CAD build for the part. Positions are in the model's coordinates, mm. A direction names the side the tool comes from. Give positions to 0.01 mm unless a question says otherwise; leave off trailing zeros. Loops run counter-clockwise (first coordinate to the right, second up) from the corner with the lowest first, then second, coordinate; pieces in that order, holes last.
```python
from build123d import *

# Parameters (mm, degrees)
RESSALTO_EXTRUS_O1_DEPTH = 6
CORTE_EXTRUS_O1_DEPTH    = 3.1
ESBO_O4_R                = 15
CORTE_EXTRUS_O2_DEPTH    = 100.844211363
ESBO_O6_R                = 2
CORTE_EXTRUS_O3_DEPTH    = 3.1
CORTE_EXTRUS_O7_DEPTH    = 10


with BuildPart() as part:
    # Esboço2 → Ressalto-extrusão1 (new body)
    with BuildSketch(Plane.XY):
        Polygon((70.472925804, 27.825776133), (30.15608873, 69.507678721), (-27.825776133, 70.472925804), (-69.507678721, 30.15608873), (-70.472925804, -27.825776133), (-30.15608873, -69.507678721), (27.825776133, -70.472925804), (69.507678721, -30.15608873), align=None)
    extrude(amount=RESSALTO_EXTRUS_O1_DEPTH)

    # Esboço3 → Corte-extrusão1 (cut)
    with BuildSketch(Plane.XY.offset(6)):
        Polygon((-61.0871998, -37.529288249), (-39.534791939, -59.811427182), (-25.159218434, -45.906647917), (-46.711626295, -23.624508984), align=None)
        Polygon((46.71864909, 23.617248408), (25.166241229, 45.899387341), (39.541814734, 59.804166606), (61.094222595, 37.522027673), align=None)
        Polygon((-59.804166606, 39.541814734), (-37.522027673, 61.094222595), (-23.617248408, 46.71864909), (-45.899387341, 25.166241229), align=None)
        Polygon((23.631531779, -46.718886871), (45.913670712, -25.16647901), (59.818449977, -39.542052515), (37.536311044, -61.094460376), align=None)
    extrude(amount=-CORTE_EXTRUS_O1_DEPTH, mode=Mode.SUBTRACT)

    # Esboço4 → Corte-extrusão2 (cut, through all)
    with BuildSketch(Plane.XY.offset(6)):
        Circle(ESBO_O4_R)
    extrude(amount=-CORTE_EXTRUS_O2_DEPTH, mode=Mode.SUBTRACT)

    # Esboço6 → Corte-extrusão3 (cut)
    with BuildSketch(Plane.XY.offset(2.9)):
        with Locations((-46.481705373, -31.053986514)):
            Circle(ESBO_O6_R)
        with Locations((-53.669492126, -38.006376147)):
            Circle(ESBO_O6_R)
        with Locations((-39.764712861, -52.381949652)):
            Circle(ESBO_O6_R)
        with Locations((-32.576926108, -45.429560019)):
            Circle(ESBO_O6_R)
        with Locations((39.779293109, 52.368949317)):
            Circle(ESBO_O6_R)
        with Locations((32.590503175, 45.417596982)):
            Circle(ESBO_O6_R)
        with Locations((53.681997779, 37.991369449)):
            Circle(ESBO_O6_R)
        with Locations((46.493207845, 31.040017114)):
            Circle(ESBO_O6_R)
        with Locations((38.006376147, -53.669492126)):
            Circle(ESBO_O6_R)
        with Locations((31.061009309, -46.488965949)):
            Circle(ESBO_O6_R)
        with Locations((52.381949652, -39.764712861)):
            Circle(ESBO_O6_R)
        with Locations((45.436582814, -32.584186684)):
            Circle(ESBO_O6_R)
        with Locations((-37.991369449, 53.681997779)):
            Circle(ESBO_O6_R)
        with Locations((-31.047038861, 46.500469435)):
            Circle(ESBO_O6_R)
        with Locations((-45.424618729, 32.597764765)):
            Circle(ESBO_O6_R)
        with Locations((-52.368949317, 39.779293109)):
            Circle(ESBO_O6_R)
    extrude(amount=-CORTE_EXTRUS_O3_DEPTH, mode=Mode.SUBTRACT)

    # Esboço7 → Corte-extrusão7 (cut)
    with BuildSketch(Plane.XY.offset(6)):
        Polygon((10.173878015, -33.609114275), (1.688596641, -25.123832901), (17.952052608, -8.860376934), (26.437333982, -17.345658308), align=None)
    extrude(amount=-CORTE_EXTRUS_O7_DEPTH, mode=Mode.SUBTRACT)


solid = part.part
```
1. Tool access for faces 4 (the face through (54.01, 30.67, 4.47)), 5 (the face through (42, -43, 2.9)), 6 (the face through (22.135, -13.044, 3.042)): list every direction of +Z, -Z, +X, -X, +Y, -Y with a clear straight run to the whole face (end or side of a thin tool).
Responses:
face 4: +Z, +Y
face 5: +Z
face 6: +Z, -Z
2. Drop flat-ended pins along their axis: pin 1 (4.5 mm diameter, centred on x = -46.48, y = -31.05, fed in from +Z); pin 2 (3 mm diameter, centred on x = 3.5, y = 11, fed in from +Z); pin 3 (2 mm diameter, centred on x = 52.5, z = 3, fed in from +Y). Give the stop position or say it passes through.
Responses:
pin 1: stops at z = 2.9
pin 2: passes through
pin 3: stops at y = 47.44
3. Saw through at C-C, the plane x = 0. List the corners of the cut face in (y, z), and give its area (3 significant figures).
Responses:
outline: (-70.01, 0) - (-15, 0) - (-15, 6) - (-70.01, 6) - close; (15, 0) - (70.01, 0) - (70.01, 6) - (15, 6) - close
area: 660 mm2
4. Pull direction X, two halves, no side cores. Call faces 1 (the face through (48.37, -50.6, 2.29)), 2 (the face through (34.62, -36.09, 4.47)), 3 (the face through (-1, 17, 0)): released by +X, released by -X, zero draft, split by the parting line, or undercut.
Responses:
face 1: released by +X
face 2: undercut
face 3: zero draft
5. Saw through at B-B, the plane y = -20. List the corners of the cut face in (x, z), and give its area (3 significant figures).
Responses:
outline: (-70.34, 0) - (6.81, 0) - (6.81, 6) - (-70.34, 6) - close; (23.78, 0) - (69.68, 0) - (69.68, 6) - (23.78, 6) - close
area: 738 mm2
6. Probe line 1 along X through (y, z) = (-25, 3.5); line 2 along Y through (x, z) = (13, 2.5); line 3 along Y through (x, z) = (-31.5, 3). List the from-to ranges inside material, lowest first.
Responses:
line 1: x = -70.43 to -48.13, -45.38 to 1.81, 18.78 to 69.59
line 2: y = -70.23 to -30.78, -13.81 to -7.48, 7.48 to 69.79
line 3: y = -68.12 to -52.04, -39.35 to 39.09, 54.87 to 66.92
7. Saw through at A-A, the plane z = 5. Count the separate pieces of the cut face and the enclosed holes in it, and give its area (3 significant figures).
Responses:
separate pieces: 1
enclosed holes: 2
area: 12,800 mm2
